Part model, mm, in its own coordinate system. Face numbers are marked on the shaded views. A direction names the side the tool comes from. Round coordinates to 2 decimals unless told otherwise and drop trailing zeros. Write each loop counter-clockwise with the first axis right and the second up, starting at its lowest first coordinate (ties: lowest second). Pieces come first, ordered by that corner, then holes. Notation, with made-up numbers: M 53.5,59.5 L 71.5,59.5 A21 cw 71.5,93.5 Z; hole C 10.5,-18.75 d11. An arc over 180 degrees is marked long. Use one line per item in the form item = value. Start each with the question number.
Item 1: Cut at A-A, the plane y = 27.5. Give the cut face in (x, z).
Item 2: Cut at B-B, the plane z = 0. Give the cut face in (x, y).
Item 3: Probe L1, parallel to X at y = 43, z = 15; L2, parallel to Y at x = 13, z = 0.5; L3, parallel to X at y = 63, z = 0. List the from-to ranges inside material, lowest first.
Item 4: Cut at C-C, the plane x = 0. Give the cut face in (y, z), then the cut area to 3 significant figures.
Item 5: Cut at D-D, the plane z = 9.5. Give the cut face in (x, y), then the cut area to 3 significant figures.
Item 6: Which spindle directions (+Z, -Z, +X, -X, +Y, -Y) get a long thin tool onto all of the face, cutting with end or side? Do the marked faces 1 and 2. Say none if no direction does.
Item 7: Flat gauge pins, fed straight in: pin 1 Ø4 at (x, z) = (15.5, 15.5) entering from +Y; pin 2 Ø12 at (x, z) = (13, -7.5) entering from +Y; pin 3 Ø0.9 at (x, z) = (15.5, 15) entering from +Y. Where does each tip first touch, or does it go through?
from build123d import *

# Parameters (mm, degrees)
EXTRUDE_1_DEPTH     = 45
SKETCH_2_R          = 11
EXTRUDE_2_DEPTH     = 2
SKETCH_3_R          = 2.5
EXTRUDE_3_DEPTH     = 23
SKETCH_4_R          = 1.55
CUT_EXTRUDE_1_DEPTH = 5


with BuildPart() as part:
    # 草图1 → 凸台-拉伸1 (new body)
    with BuildSketch(Plane(origin=(0, 0, 0), x_dir=(1, 0, 0), z_dir=(0, 1, 0))):
        Polygon((-16, 21), (-21, 16), (-21, -16), (-16, -21), (16, -21), (21, -16), (21, 16), (16, 21), align=None)
    extrude(amount=EXTRUDE_1_DEPTH)

    # 草图2 → 凸台-拉伸2 (add)
    with BuildSketch(Plane(origin=(0, 45, 0), x_dir=(1, 0, 0), z_dir=(0, 1, 0))):
        with Locations(Location((0, 0, 0), (0, 0, 270))):
            Circle(SKETCH_2_R)
    extrude(amount=EXTRUDE_2_DEPTH)

    # 草图3 → 凸台-拉伸3 (add)
    with BuildSketch(Plane(origin=(0, 47, 0), x_dir=(1, 0, 0), z_dir=(0, 1, 0))):
        with Locations(Location((0, 0, 0), (0, 0, 270))):
            Circle(SKETCH_3_R)
    extrude(amount=EXTRUDE_3_DEPTH)

    # 草图4 → 切除-拉伸1 (cut)
    with BuildSketch(Plane(origin=(0, 45, 0), x_dir=(1, 0, 0), z_dir=(0, 1, 0))):
        with Locations(Location((-15.5, 15.5, 0), (0, 0, 270))):
            Circle(SKETCH_4_R)
        with Locations(Location((15.5, 15.5, 0), (0, 0, 270))):
            Circle(SKETCH_4_R)
        with Locations(Location((-15.5, -15.5, 0), (0, 0, 270))):
            Circle(SKETCH_4_R)
        with Locations(Location((15.5, -15.5, 0), (0, 0, 270))):
            Circle(SKETCH_4_R)
    extrude(amount=-CUT_EXTRUDE_1_DEPTH, mode=Mode.SUBTRACT)


solid = part.part
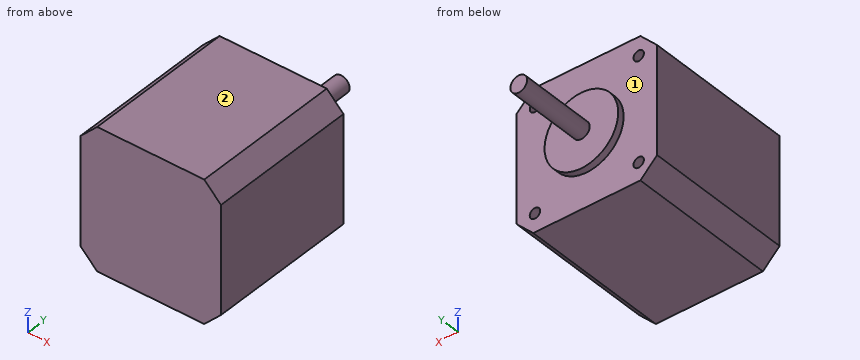
Model answer:
q1.outline = M -21,-16 L -16,-21 L 16,-21 L 21,-16 L 21,16 L 16,21 L -16,21 L -21,16 Z
q2.outline = M -21,0 L 21,0 L 21,45 L 11,45 L 11,47 L 2.5,47 L 2.5,70 L -2.5,70 L -2.5,47 L -11,47 L -11,45 L -21,45 Z
q3.L1 = -21 to -16.97, -14.03 to 14.03, 16.97 to 21
q3.L2 = 0 to 45
q3.L3 = -2.5 to 2.5
q4.outline = M 0,-21 L 45,-21 L 45,-11 L 47,-11 L 47,-2.5 L 70,-2.5 L 70,2.5 L 47,2.5 L 47,11 L 45,11 L 45,21 L 0,21 Z
q4.area = 2,050 mm²
q5.outline = M -21,0 L 21,0 L 21,45 L 5.55,45 L 5.55,47 L -5.55,47 L -5.55,45 L -21,45 Z
q5.area = 1,910 mm²
q6.face_1 = +Y
q6.face_2 = +Z, +X, -X, +Y, -Y
q7.pin_1 = 45
q7.pin_2 = 47
q7.pin_3 = 40
